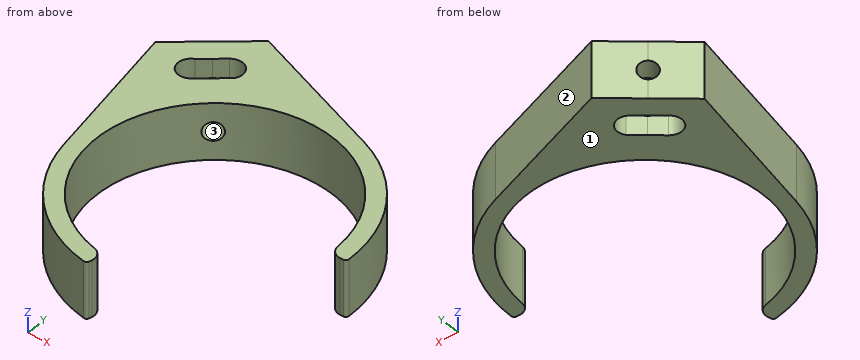
from build123d import *

# Parameters (mm, degrees)
F1_DEPTH = 25
F2_R     = 4.1301818337
F3_DEPTH = 100


with BuildPart() as f1:
    # F0 (on Top) → F1 (new body)
    with BuildSketch(Plane.XY):
        with BuildLine():
            ThreePointArc((-11.8732422152, -51.317779651), (-34.5382601184, 39.7692969136), (52.4750916265, 4.5665246966))
            ThreePointArc((52.4750916265, 4.5665246966), (54.0774628024, 1.3143944516), (57.4562661026, 0))
            Line((57.4562661026, 0), (58.8832582744, 0))
            ThreePointArc((58.8832582744, 0), (59.8641668401, 0.4130116778), (60.2542282129, 1.4032704246))
            ThreePointArc((60.2542282129, 1.4032704246), (48.9422337618, 35.1738388554), (20.5405661504, 56.662389004))
            ThreePointArc((20.5405661504, 56.662389004), (-0.9722097104, 60.2627247451), (-22.357653118, 55.9703183167))
            ThreePointArc((-22.357653118, 55.9703183167), (-39.5197577392, 45.5052736905), (-52.2859987864, 29.978584295))
            ThreePointArc((-52.2859987864, 29.978584295), (-59.5321694387, 9.4054232943), (-58.9812803638, -12.3995867702))
            ThreePointArc((-58.9812803638, -12.3995867702), (-41.7155504969, -43.5011957555), (-9.9179813794, -59.4489262374))
            ThreePointArc((-9.9179813794, -59.4489262374), (-8.9185295501, -59.2284594054), (-8.3500885012, -58.3773516818))
            Line((-8.3500885012, -58.3773516818), (-8.1064542321, -57.2139043997))
            ThreePointArc((-8.1064542321, -57.2139043997), (-8.786764538, -53.4972420783), (-11.8732422152, -51.317779651))
        make_face()
        with BuildLine():
            ThreePointArc((-22.357653118, 55.9703183167), (-0.9722097104, 60.2627247451), (20.5405661504, 56.662389004))
            Line((20.5405661504, 56.662389004), (-42.9458399328, 79.6767155568))
            Line((-42.9458399328, 79.6767155568), (-22.357653118, 55.9703183167))
        make_face()
        with BuildLine():
            Line((-72.8741856011, 53.6849815351), (-58.9812803638, -12.3995867702))
            ThreePointArc((-58.9812803638, -12.3995867702), (-59.5321694387, 9.4054232943), (-52.2859987864, 29.978584295))
            Line((-52.2859987864, 29.978584295), (-72.8741856011, 53.6849815351))
        make_face()
        with BuildLine():
            ThreePointArc((-52.2859987864, 29.978584295), (-39.5197577392, 45.5052736905), (-22.357653118, 55.9703183167))
            Line((-22.357653118, 55.9703183167), (-42.9458399328, 79.6767155568))
            Line((-42.9458399328, 79.6767155568), (-57.910012767, 66.680848546))
            Line((-57.910012767, 66.680848546), (-72.8741856011, 53.6849815351))
            Line((-72.8741856011, 53.6849815351), (-52.2859987864, 29.978584295))
        make_face()
        with BuildLine():
            Line((-55.9134628832, 55.172447865), (-51.3541472465, 59.1320559457))
            Line((-51.3541472465, 59.1320559457), (-46.7948316098, 63.0916640263))
            ThreePointArc((-46.7948316098, 63.0916640263), (-39.210764144, 63.0457975526), (-38.2846281265, 55.5183507652))
            Line((-38.2846281265, 55.5183507652), (-43.9458746166, 50.6017538162))
            Line((-43.9458746166, 50.6017538162), (-49.6071211066, 45.6851568672))
            ThreePointArc((-49.6071211066, 45.6851568672), (-58.1561290716, 46.8421101497), (-55.9134628832, 55.172447865))
        make_face(mode=Mode.SUBTRACT)
    extrude(amount=F1_DEPTH)

    # F2 (on face) → F3 (cut)
    with BuildSketch(Plane(origin=(-57.910012767, 66.680848546, 0), x_dir=(-0.7550165253, -0.6557057622, 0), z_dir=(-0.6557057622, 0.7550165253, 0))):
        with Locations((0, 12.5)):
            Circle(F2_R)
    extrude(amount=-F3_DEPTH, mode=Mode.SUBTRACT)


solid = f1.part
Geometry: final body of the model. Coordinates: model frame, mm. Face numbers are marked on the shaded views. Give positions to 0.01 mm unless a question says otherwise; leave off trailing zeros. Write each loop counter-clockwise with the first axis right and the second up, starting at its lowest first coordinate (ties: lowest second). Pieces come first, ordered by that corner, then holes. Notation, with made-up numbers: (68, 81.5) -> (125, 81.5) arc R19 ccw to (125, 101.5) -> close; hole circle Ø11 at (-32.75, 57). An arc over 180 degrees is marked (long way). Answer in a Markdown table with one row per item.
(1) Pin query (flat end, axial travel): pin 1 (4 mm diameter, centred on x = -52.5, z = 9.5, fed in from +Y); pin 2 (10 mm diameter, centred on x = 5, z = 11.5, fed in from -Y); pin 3 (12 mm diameter, centred on x = -32.5, z = 20, fed in from +Y). Return the tip coordinate at first contact, or that it passes through.
Answers below:
| item | result |
|---|---|
| pin 1 | y = 73.12 |
| pin 2 | y = 51.72 |
| pin 3 | y = 78.07 |
(2) Section query A-A on z = 22.5. Return loops of the section in (x, y).
Answers below:
| item | result |
|---|---|
| outline | (-72.87, 53.68) -> (-58.98, -12.4) arc R60.27 ccw to (-9.92, -59.45) arc R1.37 ccw to (-8.35, -58.38) -> (-8.11, -57.21) arc R5 ccw to (-11.87, -51.32) arc R52.67 cw (long way) to (52.48, 4.57) arc R5 ccw to (57.46, 0) -> (58.88, 0) arc R1.37 ccw to (60.25, 1.4) arc R60.27 ccw to (20.54, 56.66) -> (-42.95, 79.68) -> close; hole (-55.91, 55.17) arc R5.74 ccw (long way) to (-49.61, 45.69) -> (-38.28, 55.52) arc R5.74 ccw to (-46.79, 63.09) -> close |
(3) Section query B-B on x = -18. Return loops of the section in (y, z), then the cut area to 3 significant figures.
Answers below:
| item | result |
|---|---|
| outline | (-57.52, 0) -> (-49.5, 0) -> (-49.5, 25) -> (-57.52, 25) -> close; (49.5, 0) -> (70.63, 0) -> (70.63, 25) -> (49.5, 25) -> close |
| area | 729 mm^2 |
(4) Draft query along Z for the marked faces 1, 2 and 3. Return one class per face: +Z half, -Z half, draft (parallel to the pull), parting line (faces both ways), or undercut.
Answers below:
| item | result |
|---|---|
| face 1 | -Z half |
| face 2 | draft |
| face 3 | undercut |
(5) Ray query, line 1 along Y through (x, z) = (-40.5, 12); line 2 along Y through (x, z) = (-13, 17.25); line 3 along Y through (x, z) = (-30, 2.75). Return the intervals inside material, ascending. Write a range as [from, to].
Answers below:
| item | result |
|---|---|
| line 1 | [-44.64, -33.68], [33.68, 40.38], [52.89, 53.59], [63.91, 78.79] |
| line 2 | [-58.85, -51.04], [51.04, 68.82] |
| line 3 | [-52.27, -43.3], [43.3, 74.98] |
(6) Section query D-D on y = -24.5. Return loops of the section in (x, z), then the cut area to 3 significant figures.
Answers below:
| item | result |
|---|---|
| outline | (-55.07, 0) -> (-46.63, 0) -> (-46.63, 25) -> (-55.07, 25) -> close |
| area | 211 mm^2 |
(7) Section query C-C on x = -40.5. State how many separate pieces and enclosed holes the cut face has, then the cut area to 3 significant figures.
Answers below:
| item | result |
|---|---|
| separate pieces | 3 |
| enclosed holes | 1 |
| area | 1,060 mm^2 |
